Build history of the part. All positions in model axes, mm. A direction names the side the tool comes from. Round coordinates to 2 decimals unless told otherwise and drop trailing zeros. Write each loop counter-clockwise with the first axis right and the second up, starting at its lowest first coordinate (ties: lowest second). Pieces come first, ordered by that corner, then holes. Notation, with made-up numbers: (-30, 41.25) - (5, 41.25) arc R13 cw to (5, 62.25) - close; hole circle Ø1 at (62, 63.25). An arc over 180 degrees is marked (long way). Answer as a JSON object with one key per item and string values. Group by question number.
Item 1: Probe line 1 (X direction, y = 257, z = 0); line 2 (Z direction, x = 154, y = 395); line 3 (Z direction, x = 0, y = 181). List the from-to ranges inside material, lowest first. Write a range as from..to.
Item 2: Slice it at A-A, the plane y = 327. List the corners of the cut face in (x, z).
Item 3: Which spindle directions (+Z, -Z, +X, -X, +Y, -Y) get a long thin tool onto all of the face, cutting with end or side? Do faces 4 (the flat face through (135, 450.01, 239)), 5 (the cylindrical face through (-277.625, 221.86, -18.773)). Say none if no direction does.
Item 4: Flat gauge pins, fed straight in: pin 1 (8 mm diameter, centred on y = 139.5, z = 284.5, fed in from -X); pin 2 (11.5 mm diameter, centred on x = 7.5, z = -7.5, fed in from +Y); pin 3 (8 mm diameter, centred on y = 192.5, z = -55.5, fed in from +X). Where does each tip first touch, or does it go through?
Item 5: Two-plate mould, pull along X, no slides. Class faces 1 (the flat face through (-16, 450.01, 11)), 2 (the cylindrical face through (223.16, 221.85, -326.49)), 3 (the cylindrical face through (20.03, 221.86, -6.31)): +X half, -X half, draft (parallel to the pull), parting line (faces both ways), or undercut.
from build123d import *

# Parameters (mm, degrees)
BOSS_EXTRUDE1_DEPTH = 0.01
SKETCH2_R           = 64.5
SKETCH2_R_2         = 62.5
SKETCH2_R_3         = 21
SKETCH2_R_4         = 19
BOSS_EXTRUDE2_DEPTH = 450


with BuildPart() as part:
    # Sketch1 → Boss-Extrude1 (new body)
    with BuildSketch(Plane(origin=(0, 0, 0), x_dir=(1, 0, 0), z_dir=(0, 1, 0))):
        with BuildLine():
            Line((-37.239092363, 64.5), (-337.239092363, 64.5))
            ThreePointArc((-337.239092363, 64.5), (-401.739092363, 0), (-337.239092363, -64.5))
            Line((-337.239092363, -64.5), (-37.239092363, -64.5))
            Line((-37.239092363, -64.5), (112.760907637, -324.307621135))
            ThreePointArc((112.760907637, -324.307621135), (200.869546181, -347.916259679), (224.478184725, -259.807621135))
            Line((224.478184725, -259.807621135), (74.478184725, 0))
            Line((74.478184725, 0), (224.478184725, 259.807621135))
            ThreePointArc((224.478184725, 259.807621135), (200.869546181, 347.916259679), (112.760907637, 324.307621135))
            Line((112.760907637, 324.307621135), (-37.239092363, 64.5))
        make_face()
    extrude(amount=BOSS_EXTRUDE1_DEPTH)

    # Sketch2 → Boss-Extrude2 (add)
    with BuildSketch(Plane(origin=(0, 0.01, 0), x_dir=(1, 0, 0), z_dir=(0, 1, 0))):
        with Locations((168.619546181, 292.057621135)):
            Circle(SKETCH2_R)
        with Locations((168.619546181, 292.057621135)):
            Circle(SKETCH2_R_2, mode=Mode.SUBTRACT)
        with Locations((-337.239092363, 0)):
            Circle(SKETCH2_R)
        with Locations((-337.239092363, 0)):
            Circle(SKETCH2_R_2, mode=Mode.SUBTRACT)
        with Locations((168.619546181, -292.057621135)):
            Circle(SKETCH2_R)
        with Locations((168.619546181, -292.057621135)):
            Circle(SKETCH2_R_2, mode=Mode.SUBTRACT)
        Circle(SKETCH2_R_3)
        Circle(SKETCH2_R_4, mode=Mode.SUBTRACT)
    extrude(amount=BOSS_EXTRUDE2_DEPTH)


solid = part.part
Geometry says:
{
 "1": {"line 1": "x = -401.74..-399.74, -274.74..-272.74, -21..-19, 19..21", "line 2": "z = -354.88..-352.82, -231.29..-229.24, 229.24..231.29, 352.82..354.88", "line 3": "z = -21..-19, 19..21"},
 "2": {"outline": "circle Ø129 at (-337.24, 0); circle Ø42 at (0, 0); circle Ø129 at (168.62, -292.06); circle Ø129 at (168.62, 292.06); hole circle Ø125 at (-337.24, 0); hole circle Ø38 at (0, 0); hole circle Ø125 at (168.62, -292.06); hole circle Ø125 at (168.62, 292.06)"},
 "3": {"face 4": "+Z, -Z, +X, -X, +Y", "face 5": "+Y"},
 "4": {"pin 1": "stops at x = 104.22", "pin 2": "stops at y = 0.01", "pin 3": "stops at x = -298.41"},
 "5": {"face 1": "draft", "face 2": "parting line", "face 3": "undercut"}
}
